from build123d import *

# Parameters (mm, degrees)
CROQUIS1_R              = 140
CROQUIS1_R_2            = 85
SALIENTE_EXTRUIR1_DEPTH = 3
CROQUIS2_R              = 4
CORTAR_EXTRUIR1_DEPTH   = 4


with BuildPart() as part:
    # Croquis1 → Saliente-Extruir1 (new body)
    with BuildSketch(Plane(origin=(0, 0, 0), x_dir=(1, 0, 0), z_dir=(0, 1, 0))):
        Circle(CROQUIS1_R)
        Circle(CROQUIS1_R_2, mode=Mode.SUBTRACT)
    extrude(amount=SALIENTE_EXTRUIR1_DEPTH)

    # Croquis2 → Cortar-Extruir1 (cut, through all)
    with BuildSketch(Plane(origin=(0, 3, 0), x_dir=(1, 0, 0), z_dir=(0, 1, 0))):
        with Locations((0, 120)):
            Circle(CROQUIS2_R)
        with Locations((103.923048454, 60)):
            Circle(CROQUIS2_R)
        with Locations((103.923048454, -60)):
            Circle(CROQUIS2_R)
        with Locations((0, -120)):
            Circle(CROQUIS2_R)
        with Locations((-103.923048454, -60)):
            Circle(CROQUIS2_R)
        with Locations((-103.923048454, 60)):
            Circle(CROQUIS2_R)
    extrude(amount=-CORTAR_EXTRUIR1_DEPTH, mode=Mode.SUBTRACT)


solid = part.part
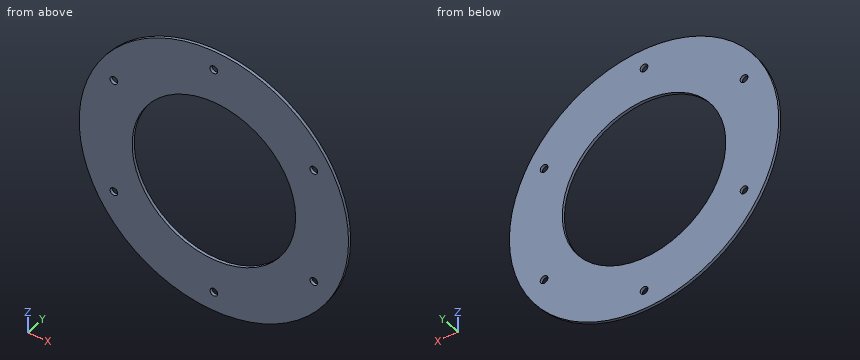
Source: CAD feature listing. Evaluate the final solid. Frame: model axes, mm. Give positions to 0.01 mm unless a question says otherwise; leave off trailing zeros. Write each loop counter-clockwise with the first axis right and the second up, starting at its lowest first coordinate (ties: lowest second). Pieces come first, ordered by that corner, then holes. Notation, with made-up numbers: M 22,-39 L 27,-39 A33 cw 27,-6 Z; hole C -40,-2 d9. An arc over 180 degrees is marked long. Answer as a JSON object with one key per item and string values.
Q1. Contact query for a flat-ended pin moving along its axis: P1, Ø5, axis at x = -103.92, z = -60, coming from the +Y side. Output: stop coordinate, or through.
Geometry check:
{"P1": "passes through"}
Q2. Cut plane B-B, the plane y = 1.3. Return the cut outline in (x, z).
Geometry check:
{"outline": "C 0,0 d280; hole C -103.92,-60 d8; hole C -103.92,60 d8; hole C 0,0 d170; hole C 0,-120 d8; hole C 0,120 d8; hole C 103.92,-60 d8; hole C 103.92,60 d8"}
Q3. Cut plane A-A, the plane x = 0. Return the cut outline in (y, z).
Geometry check:
{"outline": "M 0,-140 L 3,-140 L 3,-124 L 0,-124 Z; M 0,-116 L 3,-116 L 3,-85 L 0,-85 Z; M 0,85 L 3,85 L 3,116 L 0,116 Z; M 0,124 L 3,124 L 3,140 L 0,140 Z"}
Q4. Cut plane C-C, the plane z = 0. Return the cut outline in (x, y), then the cut area to 3 significant figures.
Geometry check:
{"outline": "M -140,0 L -85,0 L -85,3 L -140,3 Z; M 85,0 L 140,0 L 140,3 L 85,3 Z", "area": "330 mm^2"}
Q5. Cut plane D-D, the plane x = -69. Return the cut outline in (y, z), then the cut area to 3 significant figures.
Geometry check:
{"outline": "M 0,-121.82 L 3,-121.82 L 3,-49.64 L 0,-49.64 Z; M 0,49.64 L 3,49.64 L 3,121.82 L 0,121.82 Z", "area": "433 mm^2"}
Q6. Ray query, line 1 along Z through (x, y) = (0, 2.2); line 2 along X through (y, z) = (0.9, 0); line 3 along X through (y, z) = (1.4, -60). Return the intervals inside material, ascending.
Geometry check:
{"line 1": "z = -140 to -124, -116 to -85, 85 to 116, 124 to 140", "line 2": "x = -140 to -85, 85 to 140", "line 3": "x = -126.49 to -107.92, -99.92 to -60.21, 60.21 to 99.92, 107.92 to 126.49"}
